CAD build for the part. Positions are in the model's coordinates, mm. A direction names the side the tool comes from. Give positions to 0.01 mm unless a question says otherwise; leave off trailing zeros. Order: outer loops, then holes, each group sorted by start corner. A loop starts at its lowest first (then second) coordinate and runs counter-clockwise, first axis right, second up. Notation, with made-up numbers: (61.5, 36.25) -> (78.5, 36.25) arc R29 cw to (78.5, 60.25) -> close; hole circle Ø5 at (-18.75, -15). An arc over 180 degrees is marked (long way). Answer as CSV lines item,"result".
```python
from build123d import *

# Parameters (mm, degrees)
SKETCH1_R           = 65
BOSS_EXTRUDE1_DEPTH = 5
SKETCH11_R          = 4
CUT_EXTRUDE1_DEPTH  = 10
SKETCH12_R          = 30
BOSS_EXTRUDE2_DEPTH = 10
SKETCH13_R          = 22.5
CUT_EXTRUDE2_DEPTH  = 16


with BuildPart() as part:
    # Sketch1 → Boss-Extrude1 (new body)
    with BuildSketch(Plane.XY.offset(5)):
        Circle(SKETCH1_R)
    extrude(amount=-BOSS_EXTRUDE1_DEPTH)

    # Sketch11 → Cut-Extrude1 (cut)
    with BuildSketch(Plane.XY.offset(5)):
        with Locations((-25, 45)):
            Circle(SKETCH11_R)
        with Locations((25, 45)):
            Circle(SKETCH11_R)
        with Locations((26.47114317, -44.150635095)):
            Circle(SKETCH11_R)
        with Locations((51.47114317, -0.849364905)):
            Circle(SKETCH11_R)
        with Locations((-51.47114317, -0.849364905)):
            Circle(SKETCH11_R)
        with Locations((-26.47114317, -44.150635095)):
            Circle(SKETCH11_R)
    extrude(amount=-CUT_EXTRUDE1_DEPTH, mode=Mode.SUBTRACT)

    # Sketch12 → Boss-Extrude2 (add)
    with BuildSketch(Plane.XY.offset(5)):
        Circle(SKETCH12_R)
    extrude(amount=BOSS_EXTRUDE2_DEPTH)

    # Sketch13 → Cut-Extrude2 (cut, through all)
    with BuildSketch(Plane.XY.offset(15)):
        Circle(SKETCH13_R)
    extrude(amount=-CUT_EXTRUDE2_DEPTH, mode=Mode.SUBTRACT)


solid = part.part
```
1) Band-saw the part on B-B, the plane y = 15.5. Write the cut outline in (x, z).
Data:
outline,"(-63.12, 0) -> (-16.31, 0) -> (-16.31, 15) -> (-25.69, 15) -> (-25.69, 5) -> (-63.12, 5) -> close; (16.31, 0) -> (63.12, 0) -> (63.12, 5) -> (25.69, 5) -> (25.69, 15) -> (16.31, 15) -> close"
2) Pull direction Y, two halves, no side cores. Call faces 1 (the cylindrical face through (62, 19.52, 2.54)), 2 (the cylindrical face through (55.166, -2.381, 2.535)), 3 (the flat face through (28, -14, 5)): pulls with the +Y half, pulls with the -Y half, needs draft (parallel to the pull), parting line crosses it, or undercut.
Data:
face 1,"parting line crosses it"
face 2,"undercut"
face 3,"needs draft"
3) Band-saw the part on C-C, the plane x = 25. Write the cut outline in (y, z).
Data:
outline,"(-60, 0) -> (-47.87, 0) -> (-47.87, 5) -> (-60, 5) -> close; (-40.43, 0) -> (41, 0) -> (41, 5) -> (16.58, 5) -> (16.58, 15) -> (-16.58, 15) -> (-16.58, 5) -> (-40.43, 5) -> close; (49, 0) -> (60, 0) -> (60, 5) -> (49, 5) -> close"
4) Which spindle directions (+Z, -Z, +X, -X, +Y, -Y) get a long thin tool onto all of the face, cutting with end or side? Do faces 4 (the cylindrical face through (-29.97, 1.32, 9.93)), 5 (the flat face through (28, 1, 0)). Say none if no direction does.
Data:
face 4,"+Z"
face 5,"-Z, +X, -X, +Y, -Y"
5) Band-saw the part on D-D, the plane y = 45. Write the cut outline in (x, z), then the cut area to 3 significant figures.
Data:
outline,"(-46.9, 0) -> (-29, 0) -> (-29, 5) -> (-46.9, 5) -> close; (-21, 0) -> (21, 0) -> (21, 5) -> (-21, 5) -> close; (29, 0) -> (46.9, 0) -> (46.9, 5) -> (29, 5) -> close"
area,"389 mm2"
6) Band-saw the part on A-A, the plane x = 0. Write the cut outline in (y, z), then the cut area to 3 significant figures.
Data:
outline,"(-65, 0) -> (-22.5, 0) -> (-22.5, 15) -> (-30, 15) -> (-30, 5) -> (-65, 5) -> close; (22.5, 0) -> (65, 0) -> (65, 5) -> (30, 5) -> (30, 15) -> (22.5, 15) -> close"
area,"575 mm2"
7) Wall check: line 1 along Y through (x, z) = (25, 2.2); line 2 along Y through (x, z) = (-28, 3.25); line 3 along Z through (x, y) = (28.5, -27). Give the ranges that are in metal, low to high. Write a range as [from, to].
Data:
line 1,"y = [-60, -47.87], [-40.43, 41], [49, 60]"
line 2,"y = [-58.66, -47.85], [-40.45, 42.35], [47.65, 58.66]"
line 3,"z = [0, 5]"
8) Pin check, flat tips, straight feed: P1, Ø10.5, axis at x = -25, y = 45, coming from the +Z side; P2, Ø5, axis at y = 26.5, z = 9, coming from the -X side; P3, Ø6, axis at x = -10, z = 13, coming from the -Y side. Stop position of each tip, or through.
Data:
P1,"stops at z = 5"
P2,"stops at x = -18"
P3,"stops at y = -29.17"
